Model file for the job. Use its own axes, mm. Give positions to 0.01 mm unless a question says otherwise; leave off trailing zeros. Order: outer loops, then holes, each group sorted by start corner. A loop starts at its lowest first (then second) coordinate and runs counter-clockwise, first axis right, second up. Notation, with made-up numbers: (38.5, 12) -> (87.5, 12) arc R20 cw to (87.5, 44) -> close; hole circle Ø4 at (45, 73.5). An arc over 180 degrees is marked (long way). Use CSV: the item, a comma, the result in double quotes. Start each with the question number.
1. Drop flat-ended pins along their axis: pin 1 (6 mm diameter, centred on x = 4, z = 51.5, fed in from -Y); pin 2 (11 mm diameter, centred on x = -2.5, y = 0.5, fed in from -Z); pin 3 (1.5 mm diameter, centred on x = 6.5, z = 24.5, fed in from -Y); pin 4 (1 mm diameter, centred on x = -6, y = 4, fed in from -Z). Give the stop position or say it passes through.
2. Wall check: line 1 (Y direction, x = 0, z = 167.5); line 2 (Z direction, x = -1, y = -8.75); line 3 (Y direction, x = -3, z = 121). Give the ranges that are in metal, low to high. Write a range as from..to.
3. Cut at A-A on z = 104.5. List the corners of the cut face in (x, y).
```python
from build123d import *

# Parameters (mm, degrees)
CHAMFER_1_SIZE = 2
CHAMFER_2_SIZE = 0.5


with BuildPart() as part:
    # Эскиз1 → Повернуть1 (revolve)
    with BuildSketch(Plane(origin=(0, 0, 0), x_dir=(0, 0, -1), z_dir=(1, 0, 0)), mode=Mode.PRIVATE) as revolve_1_sk:
        Polygon((0, 0), (0, 5.1), (-175, 5.1), (-175, 7.5), (-179, 7.5), (-179, 10), (-183, 10), (-183, 3.05), (-143, 3.05), (-140.777028701, 0), align=None)
    revolve(revolve_1_sk.sketch.rotate(Axis((0, 0, 0), (0, 0, 1)), 90), axis=Axis((0, 0, 0), (0, 0, 1)))  # turned: the seam where the file's is

    # Фаска1
    chamfer_1_edges = [part.edges().sort_by_distance(p)[0] for p in [
        (5.1, 0, 0),
        (3.05, 0, 183),
    ]]
    chamfer(chamfer_1_edges, length=CHAMFER_1_SIZE)

    # Фаска2
    chamfer_2_edges = [part.edges().sort_by_distance(p)[0] for p in [
        (10, 0, 183),
        (10, 0, 179),
        (7.5, 0, 175),
    ]]
    chamfer(chamfer_2_edges, length=CHAMFER_2_SIZE)


solid = part.part
```
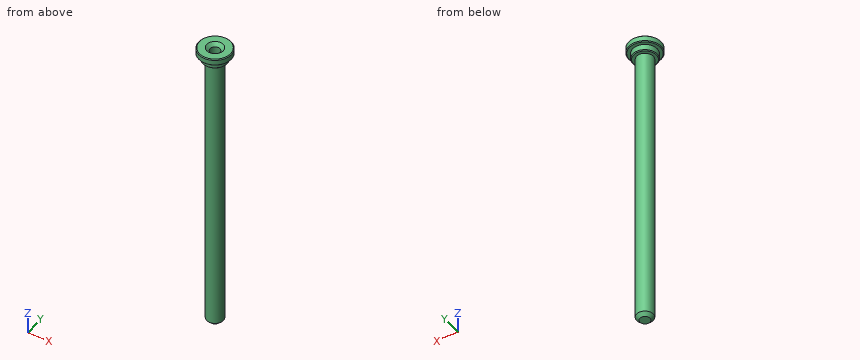
Verdict:
1,pin 1,"y = -5"
1,pin 2,"z = 0"
1,pin 3,"through"
1,pin 4,"z = 175"
2,line 1,"-5.1..-3.05, 3.05..5.1"
2,line 2,"179..183"
2,line 3,"-4.12..4.12"
3,outline,"circle Ø10.2 at (0, 0)"
